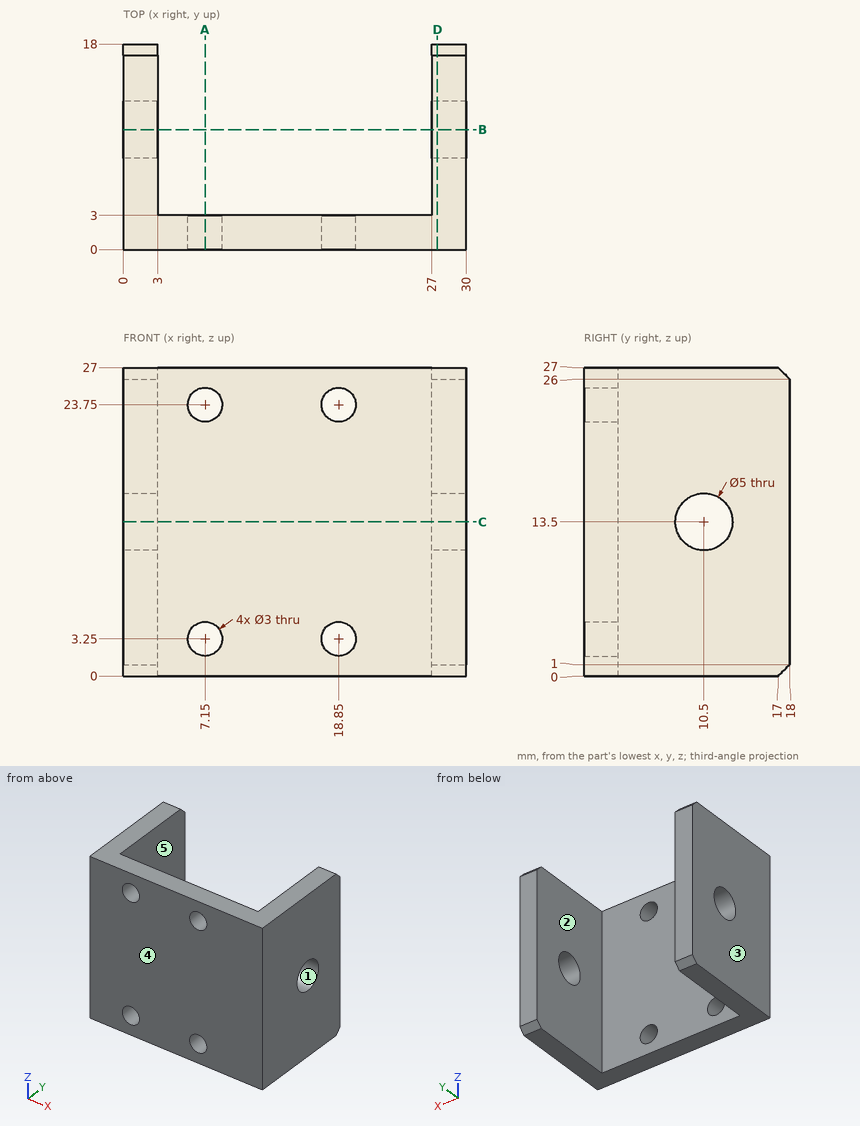
Verification items for this drawing (mm, ordinates from the low corner). A direction names the side the tool comes from. Give positions to 0.01 mm unless a question says otherwise; leave off trailing zeros. Write each loop counter-clockwise with the first axis right and the second up, starting at its lowest first coordinate (ties: lowest second). Pieces come first, ordered by that corner, then holes.
1) Material ranges on L1, parallel to Z at x = 7.15, y = 1.3; L2, parallel to X at y = 1.2, z = 23.75; L3, parallel to X at y = 16, z = 4.5, recorded low to high.
2) Section check D-D, the plane x = 27.5. Record the boundary of the cut face in (y, z), and give its area (3 significant figures).
3) Access from +Z, -Z, +X, -X, +Y, -Y to the whole of each face (thin tool, end or side, straight path). Record for the marked faces 4 and 5.
4) Section check C-C, the plane z = 13.5. Record the boundary of the cut face in (x, y).
5) Gauge pin test, flat ends, axial feed: pin 1 (1.5 mm diameter, centred on y = 11, z = 11.5, fed in from +X); pin 2 (4 mm diameter, centred on x = 18.85, z = 23.75, fed in from +Y); pin 3 (4.5 mm diameter, centred on y = 10.5, z = 13.5, fed in from +X). Record the tip position at first contact, or that the pin passes through.
6) Section check B-B, the plane y = 10.5. Record the boundary of the cut face in (x, z).
7) Section check A-A, the plane x = 7.15. Record the boundary of the cut face in (y, z).
8) Release check for a two-part mould opening along X. For the marked faces 1, 2 and 3 record: pulls with the +X half, pulls with the -X half, needs draft (parallel to the pull), parting line crosses it, or undercut.
Computed:
1. L1: z = 0 to 1.75, 4.75 to 22.25, 25.25 to 27
1. L2: x = 0 to 5.65, 8.65 to 17.35, 20.35 to 30
1. L3: x = 0 to 3, 27 to 30
2. outline: (0, 0) - (17, 0) - (18, 1) - (18, 26) - (17, 27) - (0, 27) - close; hole circle Ø5 at (10.5, 13.5)
2. area: 465 mm2
3. face 4: +Z, -Z, +X, -X, -Y
3. face 5: +Z, -Z, +Y
4. outline: (0, 0) - (30, 0) - (30, 8) - (27, 8) - (27, 3) - (3, 3) - (3, 8) - (0, 8) - close; (0, 13) - (3, 13) - (3, 18) - (0, 18) - close; (27, 13) - (30, 13) - (30, 18) - (27, 18) - close
5. pin 1: stops at x = 30
5. pin 2: stops at y = 3
5. pin 3: passes through
6. outline: (0, 0) - (3, 0) - (3, 11) - (0, 11) - close; (0, 16) - (3, 16) - (3, 27) - (0, 27) - close; (27, 0) - (30, 0) - (30, 11) - (27, 11) - close; (27, 16) - (30, 16) - (30, 27) - (27, 27) - close
7. outline: (0, 0) - (3, 0) - (3, 1.75) - (0, 1.75) - close; (0, 4.75) - (3, 4.75) - (3, 22.25) - (0, 22.25) - close; (0, 25.25) - (3, 25.25) - (3, 27) - (0, 27) - close
8. face 1: needs draft
8. face 2: undercut
8. face 3: pulls with the -X half
